Design review of the part built by this model. Coordinates are the model's own, in mm. Face numbers are marked on the shaded views. A direction names the side the tool comes from. Coordinates: 2 decimals unless noted, no trailing zeros. Order: outer loops, then holes, each group sorted by start corner. A loop starts at its lowest first (then second) coordinate and runs counter-clockwise, first axis right, second up.
from build123d import *

# Parameters (mm, degrees)
SKETCH_1_R          = 10
SKETCH_1_R_2        = 1.9
SKETCH_1_R_3        = 2
EXTRUDE_6_DEPTH     = 20
SKETCH_12_R         = 11.5
SKETCH_12_R_2       = 3.1
EXTRUDE_8_DEPTH     = 4
SKETCH_13_R         = 3
CUT_EXTRUDE_7_DEPTH = 2
FILLET_3_R          = 2
CUT_EXTRUDE_START   = -4
SKETCH_14_R         = 10
CUT_EXTRUDE_8_DEPTH = 4
SKETCH_15_R         = 3.25
CUT_EXTRUDE_9_DEPTH = 3


with BuildPart() as part:
    # 草图1 → 凸台-拉伸6 (new body)
    with BuildSketch(Plane(origin=(0, 0, 0), x_dir=(1, 0, 0), z_dir=(0, 1, 0))):
        with Locations(Location((0, 0, 0), (0, 0, 270))):
            Circle(SKETCH_1_R)
        with Locations(Location((-5, 5, 0), (0, 0, 270))):
            Circle(SKETCH_1_R_2, mode=Mode.SUBTRACT)
        with Locations(Location((5, 5, 0), (0, 0, 270))):
            Circle(SKETCH_1_R_2, mode=Mode.SUBTRACT)
        with Locations(Location((5, -5, 0), (0, 0, 270))):
            Circle(SKETCH_1_R_2, mode=Mode.SUBTRACT)
        with Locations(Location((-5, -5, 0), (0, 0, 270))):
            Circle(SKETCH_1_R_2, mode=Mode.SUBTRACT)
        with Locations(Location((0, 0, 0), (0, 0, 270))):
            Circle(SKETCH_1_R_3, mode=Mode.SUBTRACT)
    extrude(amount=EXTRUDE_6_DEPTH)

    # 草图12 → 凸台-拉伸8 (add)
    with BuildSketch(Plane.XZ):
        with Locations(Location((0, 0, 0), (0, 0, 270))):
            Circle(SKETCH_12_R)
        Circle(SKETCH_12_R_2, mode=Mode.SUBTRACT)
    extrude(amount=-EXTRUDE_8_DEPTH)

    # 草图13 → 切除-拉伸7 (cut)
    with BuildSketch(Plane.XZ):
        with Locations(Location((0, 0, 0), (0, 0, 270))):
            Circle(SKETCH_13_R)
    extrude(amount=-CUT_EXTRUDE_7_DEPTH, mode=Mode.SUBTRACT)

    # 圆角3
    # the kernel refuses this fillet: 2 mm, written as the material it adds along each edge
    with BuildSketch(Plane(origin=(0, 4, 0), x_dir=(0, 0, 1), z_dir=(1, 0, 0))) as fillet_3_piece_1:
        with BuildLine():
            CenterArc((12, -1.936491673), FILLET_3_R, 104.477512186, 75.522487814)
            Line((10, -1.936491673), (9.96, -1.936491673))
            Line((9.96, -1.936491673), (9.96, 0))
            Line((9.96, 0), (10, 0.04))
            ThreePointArc((10, 0.04), (10.75, 0.04), (11.49, 0.038729833))
            Line((11.49, 0.038729833), (11.5, 0))
        make_face()
    revolve(axis=Axis((0, 4, 0), (0, -1, 0)))

    # 草图14 → 切除-拉伸8 (cut)
    with BuildSketch(Plane(origin=(0, 20, 0), x_dir=(1, 0, 0), z_dir=(0, 1, 0)).offset(CUT_EXTRUDE_START)):
        with Locations(Location((0, 0, 0), (0, 0, 90))):
            Circle(SKETCH_14_R)
    extrude(amount=CUT_EXTRUDE_8_DEPTH, mode=Mode.SUBTRACT)

    # 草图15 → 切除-拉伸9 (cut)
    with BuildSketch(Plane.XZ):
        with Locations(Location((0, 0, 0), (0, 0, 270))):
            Circle(SKETCH_15_R)
    extrude(amount=-CUT_EXTRUDE_9_DEPTH, mode=Mode.SUBTRACT)


solid = part.part
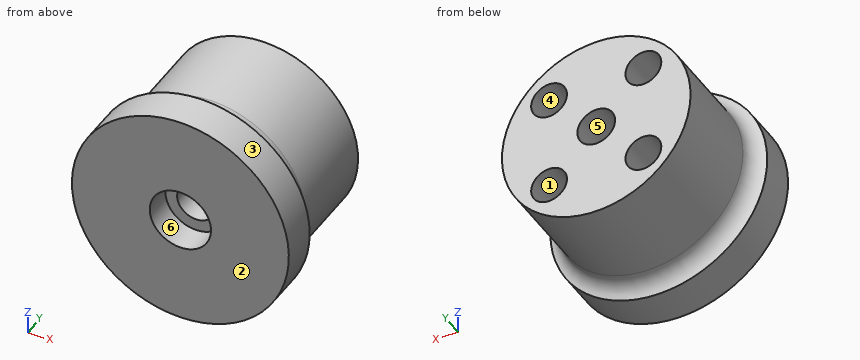
1. Add section C-C (y = 2). Give the boundary of the cut face in (x, z), and give its area (3 significant figures).
2. Add section A-A (z = 0). Give the boundary of the cut face in (x, y).
3. For the marked faces 4, 5 and 6, list the 3-axis set-ups (+Z, -Z, +X, -X, +Y, -Y) from which the entire face can be reached by the end or side of a thin tool; tool diameter is ignored.
4. Mouldability with a two-part tool opening along X and no side actions: class the marked faces 1, 2 and 3 as pulls with the +X half, pulls with the -X half, needs draft (parallel to the pull), parting line crosses it, or undercut.
5. Insertion check: pin 1 (5 mm diameter, centred on x = 0, z = 0, fed in from -Y); pin 2 (1.9 mm diameter, centred on x = 5, z = -5, fed in from +Y); pin 3 (1 mm diameter, centred on y = 8, z = 8, fed in from +X). Each pin has a flat end and moves straight along its axis. Give the tip position at first contact, or say it passes through.
6. To check wall thickness, follow line 1 (X direction, y = 12.5, z = -5.75); line 2 (X direction, y = 13.75, z = -5). State the ranges of each line that lie inside material, in increasing order.
7. Add section B-B (y = 14.25). Give the boundary of the cut face in (x, z), and give its area (3 significant figures).
Solution:
1. outline: circle Ø23 at (0, 0); hole circle Ø6.5 at (0, 0)
1. area: 382 mm2
2. outline: (-11.5, 0) - (-3.25, 0) - (-3.25, 3) - (-2, 3) - (-2, 16) - (-10, 16) - (-10, 5.94) arc R2 cw to (-11.5, 4) - close; (2, 3) - (3.25, 3) - (3.25, 0) - (11.5, 0) - (11.5, 4) arc R2 cw to (10, 5.94) - (10, 16) - (2, 16) - close
3. face 4: +Y
3. face 5: +Y, -Y
3. face 6: -Y
4. face 1: undercut
4. face 2: needs draft
4. face 3: parting line crosses it
5. pin 1: stops at y = 3
5. pin 2: stops at y = 4
5. pin 3: stops at x = 6.61
6. line 1: x = -8.18 to -6.75, -3.25 to 3.25, 6.75 to 8.18
6. line 2: x = -8.66 to -6.9, -3.1 to 3.1, 6.9 to 8.66
7. outline: circle Ø20 at (0, 0); hole circle Ø3.8 at (-5, -5); hole circle Ø3.8 at (-5, 5); hole circle Ø4 at (0, 0); hole circle Ø3.8 at (5, -5); hole circle Ø3.8 at (5, 5)
7. area: 256 mm2
